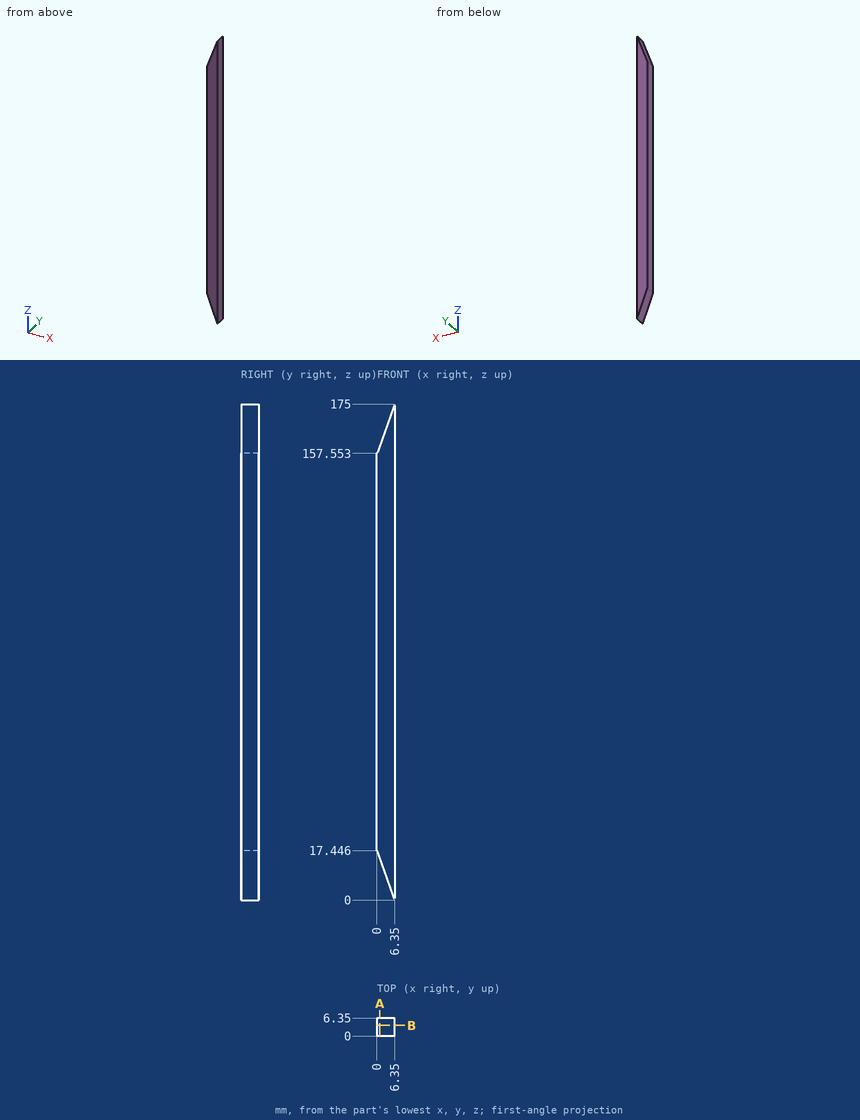
Study the drawing (mm; zero at the part's minimum x, y, z) and answer. Give positions to 0.01 mm unless a question says otherwise; leave off trailing zeros. Write each loop counter-clockwise with the first axis right and the second up, starting at its lowest first coordinate (ties: lowest second). Pieces come first, ordered by that corner, then holes. Notation, with made-up numbers: (-16.5, -30.5) -> (9.5, -30.5) arc R21 ccw to (9.5, 2.5) -> close; hole circle Ø10 at (67, 56). An arc over 180 degrees is marked (long way). Write item = value, one per line.
Q1. Section A-A on x = 1 is taken. Determine the outline of the cut face in (y, z).
Computed values:
outline = (0, 14.7) -> (6.35, 14.7) -> (6.35, 160.3) -> (0, 160.3) -> close
Q2. Consider line 1 along X through (y, z) = (6, 159.5); line 2 along X through (y, z) = (2.75, 165). Determine where each line is inside the solid, lowest interval first.
Computed values:
line_1 = 0.71 to 6.35
line_2 = 2.71 to 6.35
Q3. Section B-B on y = 3.75 is taken. Determine the outline of the cut face in (x, z), and give its area (3 significant figures).
Computed values:
outline = (0, 17.45) -> (6.35, 0) -> (6.35, 175) -> (0, 157.55) -> close
area = 1,000 mm^2
Q4. A flat-ended cylindrical pin translates along its axis: pin 1 Ø2 at (y, z) = (3.5, 65) entering from -X. Find the tip coordinate at first contact, or state that the pin passes through.
Computed values:
pin_1 = 0
